Solid Edge part; units mm, degrees
sketch "Sketch1" plane through (0, 0, 0) normal (0, 0, 1) x (1, 0, 0)
  line L0 (-44, -40) -> (44, -40)
  line L1 (44, -40) -> (44, 40)
  line L2 (44, 40) -> (-44, 40)
  line L3 (-44, 40) -> (-44, -40)
  circle A0 centre (0, 0) radius 7
  circle A1 centre (19.0919, 19.0919) radius 1.7
  circle A2 centre (-19.0919, 19.0919) radius 1.7
  circle A3 centre (-19.0919, -19.0919) radius 1.7
  circle A4 centre (19.0919, -19.0919) radius 1.7
  circle A5 centre (-20, 30) radius 1.7
  circle A6 centre (20, 30) radius 1.7
extrude "Protrusion1" add sketch "Sketch1" along normal blind 6
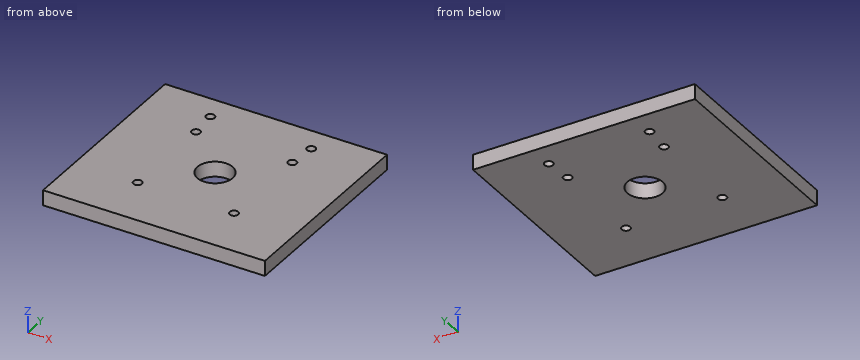
Here's how the part is built. I have some questions about the finished solid (model axes, mm). Give positions to 0.01 mm unless a question says otherwise; leave off trailing zeros. Loops run counter-clockwise (first coordinate to the right, second up) from the corner with the lowest first, then second, coordinate; pieces in that order, holes last. Notation, with made-up numbers: M 26.5,10 L 46.5,10 A30 cw 46.5,47 Z; hole C 54,68.5 d7. An arc over 180 degrees is marked long. Return JSON: item names as keys, results as strings.
Item 1: Imagine slicing it at A-A on y = 30. List the corners of the cut face in (x, z) for me, then the cut area to 3 significant figures.
A:
{"outline": "M -44,0 L -21.7,0 L -21.7,6 L -44,6 Z; M -18.3,0 L 18.3,0 L 18.3,6 L -18.3,6 Z; M 21.7,0 L 44,0 L 44,6 L 21.7,6 Z", "area": "487 mm^2"}
Item 2: Imagine slicing it at B-B on x = 0. List the corners of the cut face in (y, z) for me.
A:
{"outline": "M -40,0 L -7,0 L -7,6 L -40,6 Z; M 7,0 L 40,0 L 40,6 L 7,6 Z"}
Item 3: Please list where these lines run through material, in increasing order: line 1 (X direction, y = -19, z = 5.2); line 2 (Y direction, x = -20, z = 2.05); line 3 (X direction, y = 18.5, z = 3.3).
A:
{"line 1": "x = -44 to -20.79, -17.39 to 17.39, 20.79 to 44", "line 2": "y = -40 to -20.53, -17.65 to 17.65, 20.53 to 28.3, 31.7 to 40", "line 3": "x = -44 to -20.69, -17.5 to 17.5, 20.69 to 44"}
Item 4: Imagine slicing it at D-D on z = 2.3. List the corners of the cut face in (x, y) for me, then the cut area to 3 significant figures.
A:
{"outline": "M -44,-40 L 44,-40 L 44,40 L -44,40 Z; hole C -20,30 d3.4; hole C -19.09,-19.09 d3.4; hole C -19.09,19.09 d3.4; hole C 0,0 d14; hole C 19.09,-19.09 d3.4; hole C 19.09,19.09 d3.4; hole C 20,30 d3.4", "area": "6,830 mm^2"}
Item 5: Imagine slicing it at C-C on y = 5.5. List the corners of the cut face in (x, z) for me, then the cut area to 3 significant figures.
A:
{"outline": "M -44,0 L -4.33,0 L -4.33,6 L -44,6 Z; M 4.33,0 L 44,0 L 44,6 L 4.33,6 Z", "area": "476 mm^2"}
